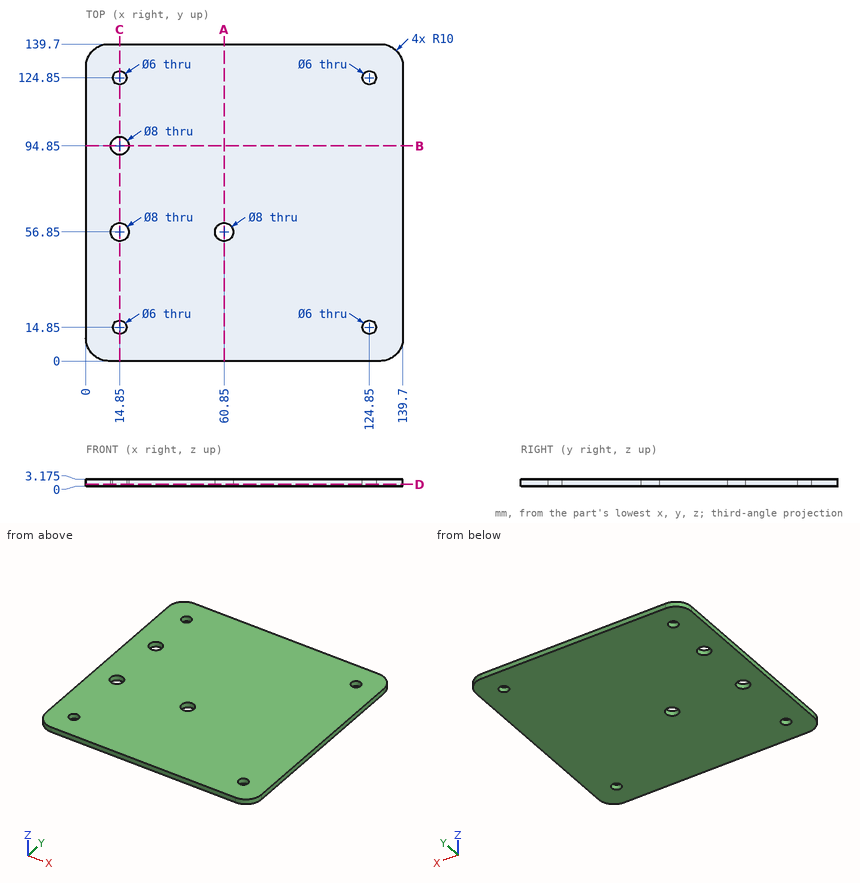
Input: dimensioned drawing with shaded views. Units: mm. Origin: part minimum x, y, z. Give positions to 0.01 mm unless a question says otherwise; leave off trailing zeros. Loops run counter-clockwise (first coordinate to the right, second up) from the corner with the lowest first, then second, coordinate; pieces in that order, holes last. Notation, with made-up numbers: (-36.5, 29) -> (-6.5, 29) arc R30 cw to (-6.5, 57) -> close; hole circle Ø6 at (-32, 67). An arc over 180 degrees is marked (long way). Return JSON: item names as keys, results as strings.
Item 1: Section C-C, the plane x = 14.85. Output: boundary loops of the cut face in (y, z) (3 decimals).
Filled in:
{"outline": "(0, 0) -> (11.85, 0) -> (11.85, 3.175) -> (0, 3.175) -> close; (17.85, 0) -> (52.85, 0) -> (52.85, 3.175) -> (17.85, 3.175) -> close; (60.85, 0) -> (90.85, 0) -> (90.85, 3.175) -> (60.85, 3.175) -> close; (98.85, 0) -> (121.85, 0) -> (121.85, 3.175) -> (98.85, 3.175) -> close; (127.85, 0) -> (139.7, 0) -> (139.7, 3.175) -> (127.85, 3.175) -> close"}
Item 2: Section D-D, the plane z = 0.85. Output: boundary loops of the cut face in (x, y), plus the area to 3 significant figures.
Filled in:
{"outline": "(0, 10) arc R10 ccw to (10, 0) -> (129.7, 0) arc R10 ccw to (139.7, 10) -> (139.7, 129.7) arc R10 ccw to (129.7, 139.7) -> (10, 139.7) arc R10 ccw to (0, 129.7) -> close; hole circle Ø8 at (14.85, 56.85); hole circle Ø8 at (14.85, 94.85); hole circle Ø6 at (14.85, 14.85); hole circle Ø6 at (14.85, 124.85); hole circle Ø8 at (60.85, 56.85); hole circle Ø6 at (124.85, 14.85); hole circle Ø6 at (124.85, 124.85)", "area": "19,200 mm^2"}
Item 3: Section B-B, the plane y = 94.85. Output: boundary loops of the cut face in (x, z) (3 decimals).
Filled in:
{"outline": "(0, 0) -> (10.85, 0) -> (10.85, 3.175) -> (0, 3.175) -> close; (18.85, 0) -> (139.7, 0) -> (139.7, 3.175) -> (18.85, 3.175) -> close"}
Item 4: Section A-A, the plane x = 60.85. Output: boundary loops of the cut face in (y, z) (3 decimals), plus the area to 3 significant figures.
Filled in:
{"outline": "(0, 0) -> (52.85, 0) -> (52.85, 3.175) -> (0, 3.175) -> close; (60.85, 0) -> (139.7, 0) -> (139.7, 3.175) -> (60.85, 3.175) -> close", "area": "418 mm^2"}
Item 5: Line query: line 1 (Y direction, x = 14.85, z = 0.85); line 2 (Y direction, x = 124.85, z = 1.75); line 3 (Y direction, x = 60.85, z = 1.3). Output: solid intervals per line, ascending.
Filled in:
{"line 1": "0 to 11.85, 17.85 to 52.85, 60.85 to 90.85, 98.85 to 121.85, 127.85 to 139.7", "line 2": "0 to 11.85, 17.85 to 121.85, 127.85 to 139.7", "line 3": "0 to 52.85, 60.85 to 139.7"}
Item 6: Pin query (flat end, axial travel): P1, Ø1.5, axis at x = 93, z = 1.5, coming from the -Y side; P2, Ø5, axis at x = 14.85, y = 56.85, coming from the -Z side. Return the tip coordinate at first contact, or that it passes through.
Filled in:
{"P1": "y = 0", "P2": "through"}
